Verification items for the finished model (mm, model axes). A direction names the side the tool comes from. Round coordinates to 2 decimals unless told otherwise and drop trailing zeros. Loops run counter-clockwise (first coordinate to the right, second up) from the corner with the lowest first, then second, coordinate; pieces in that order, holes last. Notation, with made-up numbers: (-35.75, -9) - (-9.75, -9) arc R26 ccw to (-9.75, 16) - close; hole circle Ø2 at (-18.5, 78). An arc over 180 degrees is marked (long way). Use a Markdown table: item, result. Add a question column.
Autodesk Inventor part; units mm, degrees
ref_plane "YZ Plane" through (0, 0, 0) normal (1, 0, 0) x (0, 1, 0)
ref_plane "XZ Plane" through (0, 0, 0) normal (0, 1, 0) x (-1, 0, 0)
ref_plane "XY Plane" through (0, 0, 0) normal (0, 0, 1) x (1, 0, 0)
sketch "Sketch1" plane through (0, 0, 0) normal (0, 0, 1) x (1, 0, 0)
  line L0 (-4.3779, 2.8981) -> (4.8221, 2.8981)
  line L1 (4.8221, 2.8981) -> (4.8221, -1.9019)
  line L2 (4.8221, -1.9019) -> (-4.3779, -1.9019)
  line L3 (-4.3779, -1.9019) -> (-4.3779, 2.8981)
  line L4 (-1.1779, 2.8981) -> (-1.1779, -1.9019)
  line L5 (1.6221, 2.8981) -> (1.6221, -1.9019)
  point P0 (0, 0)
  dimension "d0" = 2.8
  dimension "d1" = 9.2
  dimension "d2" = 3.2
  dimension "d11" = 4.8
extrude "Extrusion1" add sketch "Sketch1" along normal blind 4.4 contours L0 L4 L2 L3 | L0 L1 L2 L5
extrude "Extrusion2" add sketch "Sketch1" against normal blind 1
sketch "Sketch2" plane through (0, 0, -1) normal (0, 0, -1) x (-1, 0, 0)
  line L0 (4.3779, 2.8981) -> (-4.8221, 2.8981)
  line L1 (-4.8221, 2.8981) -> (-4.8221, -1.9019)
  line L2 (-4.8221, -1.9019) -> (4.3779, -1.9019)
  line L3 (4.3779, -1.9019) -> (4.3779, 2.8981)
  circle A0 centre (-3.6221, 1.7681) radius 0.25
  circle A1 centre (-3.6221, -0.7719) radius 0.25
  circle A2 centre (3.1779, 1.7681) radius 0.25
  circle A3 centre (3.1779, -0.7719) radius 0.25
  point P0 (0, 0)
  dimension "d7" = 2.54
  dimension "d8" = 6.8
  dimension "d9" = 9.2
  dimension "d10" = 4.8
  dimension "d12" = 1.13
  dimension "d13" = 1.2
  dimension "d14" = 0.5
  dimension "d15" = 0.5
  dimension "d16" = 0.5
  dimension "d17" = 0.5
extrude "Extrusion3" add sketch "Sketch2" along normal blind 2.2 contours A0 | A1 | A2 | A3
sketch "Sketch3" plane through (0, 0, 4.4) normal (0, 0, 1) x (1, 0, 0)
  line L0 (4.8221, -1.9019) -> (4.8221, 2.8981)
  line L1 (4.8221, 2.8981) -> (1.6221, 2.8981)
  line L2 (1.6221, 2.8981) -> (1.6221, -1.9019)
  line L3 (1.6221, -1.9019) -> (4.8221, -1.9019)
  line L4 (-4.3779, 2.8981) -> (-4.3779, -1.9019)
  line L5 (-4.3779, -1.9019) -> (-1.1779, -1.9019)
  line L6 (-1.1779, -1.9019) -> (-1.1779, 2.8981)
  line L7 (-1.1779, 2.8981) -> (-4.3779, 2.8981)
  line L8 (1.6221, 2.8981) -> (1.6221, -1.9019)
  line L9 (1.6221, 0.2481) -> (1.9221, 0.2481)
  line L10 (1.9221, 0.2481) -> (1.9221, 0.7481)
  line L11 (1.9221, 0.7481) -> (1.6221, 0.7481)
  line L12 (1.6221, 0.7481) -> (1.6221, 0.2481)
  line L13 (-1.1779, -0.0019) -> (-1.4779, -0.0019)
  line L14 (-1.4779, -0.0019) -> (-1.4779, 0.9981)
  line L15 (-1.4779, 0.9981) -> (-1.1779, 0.9981)
  line L16 (-1.1779, 0.9981) -> (-1.1779, -0.0019)
  point P0 (0, 0)
  dimension "d20" = 0.3
  dimension "d21" = 0.5
  dimension "d22" = 0.3
  dimension "d23" = 1
  dimension "d24" = 4.8
  dimension "d25" = 2.15
  dimension "d26" = 1.9
extrude "Extrusion4" cut sketch "Sketch3" against normal blind 2.7 contours L2 L11 L10 L9 | L6 L13 L14 L15
fillet "Fillet1" radius 0.7 4 edges at (1.6221, -1.9019, 2.2) (1.6221, 2.8981, 2.2) (-1.1779, 2.8981, 2.2) (-1.1779, -1.9019, 2.2)
fillet "Fillet1" radius 0.3 4 edges at (-4.3779, -1.9019, 1.7) (-4.3779, 2.8981, 1.7) (4.8221, 2.8981, 1.7) (4.8221, -1.9019, 1.7)
equation "\"d2\" = -0.5 * d0 + 0.5 * d1"
equation "\"d20\" = d22"
equation "\"d25\" = -0.5 * d21 + 0.5 * d24"
equation "\"d26\" = -0.5 * d23 + 0.5 * d24"
properties part number "COTS_Vishay_TCST1230_Optocoupler" material "ABS Plastic"
Q1. Section check C-C on x = 1.5. Record the cut outline in (y, z), plus the area to 3 significant figures.
Q2. Release check for a two-part mould opening along X. For faces 4 (the face through (-1.178, 1, 1)), 5 (the face through (-4.378, 0, 2)), 6 (the face through (4.822, 1, 2)), 7 (the face through (3, 1, 4.4)) record: +X half, -X half, draft (parallel to the pull), parting line (faces both ways), or undercut.
Q3. Set-up check for faces 1 (the face through (0.3, -1.902, -0.7)), 2 (the face through (-1.478, 0.5, 3.1)), 3 (the face through (1.622, 1, 2)): record each of +Z, -Z, +X, -X, +Y, -Y from which the full face is reachable in a straight line by a thin tool's end or side.
Q4. Section check D-D on z = -1.5. Record the cut outline in (x, y).
Q5. Go/stop test with a flat-tipped pin: pin 1 Ø1.5 at (y, z) = (-1.5, -2) entering from +X. Record where the tip stops, or that it passes through.
Q6. Thickness scan on line 1 along X through (y, z) = (0.6, 1.5); line 2 along Z through (x, y) = (3.5, 1.35); line 3 along Y through (x, z) = (1.75, 3.5). Record the ranges inside material, lowest first.
Q7. Section check A-A on z = 0.5. Record the cut outline in (x, y).
Q8. Section check B-B on z = 3.25. Record the cut outline in (x, y), plus the area to 3 significant figures.
Determined:
| question | item | result |
|---|---|---|
| 1 | outline | (-1.9, -1) - (2.9, -1) - (2.9, 0) - (-1.9, 0) - close |
| 1 | area | 4.80 mm² |
| 2 | face 4 | undercut |
| 2 | face 5 | -X half |
| 2 | face 6 | +X half |
| 2 | face 7 | draft |
| 3 | face 1 | +Z, -Z, +X, -X, -Y |
| 3 | face 2 | +Z |
| 3 | face 3 | +Z, +Y, -Y |
| 4 | outline | circle Ø0.5 at (-3.18, -0.77); circle Ø0.5 at (-3.18, 1.77); circle Ø0.5 at (3.62, -0.77); circle Ø0.5 at (3.62, 1.77) |
| 5 | pin 1 | stops at x = 3.87 |
| 6 | line 1 | x = -4.38 to -1.18, 1.62 to 4.82 |
| 6 | line 2 | z = -1 to 4.4 |
| 6 | line 3 | y = -1.61 to 0.25, 0.75 to 2.6 |
| 7 | outline | (-4.38, -1.6) arc R0.3 ccw to (-4.08, -1.9) - (-1.88, -1.9) arc R0.7 ccw to (-1.18, -1.2) - (-1.18, 2.2) arc R0.7 ccw to (-1.88, 2.9) - (-4.08, 2.9) arc R0.3 ccw to (-4.38, 2.6) - close; (1.62, -1.2) arc R0.7 ccw to (2.32, -1.9) - (4.52, -1.9) arc R0.3 ccw to (4.82, -1.6) - (4.82, 2.6) arc R0.3 ccw to (4.52, 2.9) - (2.32, 2.9) arc R0.7 ccw to (1.62, 2.2) - close |
| 8 | outline | (-4.38, -1.6) arc R0.3 ccw to (-4.08, -1.9) - (-1.88, -1.9) arc R0.7 ccw to (-1.18, -1.2) - (-1.18, 0) - (-1.48, 0) - (-1.48, 1) - (-1.18, 1) - (-1.18, 2.2) arc R0.7 ccw to (-1.88, 2.9) - (-4.08, 2.9) arc R0.3 ccw to (-4.38, 2.6) - close; (1.62, -1.2) arc R0.7 ccw to (2.32, -1.9) - (4.52, -1.9) arc R0.3 ccw to (4.82, -1.6) - (4.82, 2.6) arc R0.3 ccw to (4.52, 2.9) - (2.32, 2.9) arc R0.7 ccw to (1.62, 2.2) - (1.62, 0.75) - (1.92, 0.75) - (1.92, 0.25) - (1.62, 0.25) - close |
| 8 | area | 29.8 mm² |
